from build123d import *

# Parameters (mm, degrees)
F0_R      = 23.0505
F0_R_2    = 16.7005
F1_DEPTH  = 50.8
F2_R      = 23.0505
F3_DEPTH  = 25.4
F3_FACE_R = 23.0505
F4_DEPTH  = 7.62
F5_R      = 16.7005
F6_DEPTH  = 7.62


with BuildPart() as f1:
    # F0 (on Top) → F1 (new body)
    with BuildSketch(Plane.XY):
        Circle(F0_R)
        Circle(F0_R_2, mode=Mode.SUBTRACT)
    extrude(amount=F1_DEPTH)

    # F2 (on face) → F3 (join)
    with BuildSketch(Plane.XY.offset(50.8)):
        Circle(F2_R)
    extrude(amount=F3_DEPTH)

    # F3_face (on face) → F4 (join)
    with BuildSketch(Plane.XY.offset(76.2)):
        Circle(F3_FACE_R)
    extrude(amount=F4_DEPTH)

    # F5 (on face) → F6 (cut)
    with BuildSketch(Plane.XY.offset(83.82)):
        Circle(F5_R)
    extrude(amount=-F6_DEPTH, mode=Mode.SUBTRACT)


solid = f1.part
The listing builds one solid part. Answer for the finished solid, in the listing's coordinates (mm). A direction names the side the tool comes from. Give positions to 0.01 mm unless a question says otherwise; leave off trailing zeros. Write each loop counter-clockwise with the first axis right and the second up, starting at its lowest first coordinate (ties: lowest second). Pieces come first, ordered by that corner, then holes.
Item 1: Which of the six approach directions +Z, -Z, +X, -X, +Y, -Y give full straight-line access (tool end or side, diameter ignored) to faces 4 (the cylindrical face through (-3.62, -16.303, 25.044)), 5 (the cylindrical face through (-3.62, -16.303, 80.063)), 6 (the flat face through (12, 12, 0))?
Item 2: Section C-C, the plane z = 14.5 is taken. Write down the section's boundary in (x, y).
Item 3: Find the intervals of material crossed by line 1 along Y through (x, z) = (0, 79); line 2 along Z through (x, y) = (-0.5, -1); line 3 along Y through (x, z) = (-7, 38), in increasing order.
Item 4: Determine the mould class of faces 1 (the cylindrical face through (-5, -22.5, 41.3)), 2 (the flat face through (12, 12, 83.82)), 3 (the flat face through (0, 0, 50.8)) for opening direction Y: released by +Y, released by -Y, zero draft, split by the parting line, or undercut.
Item 5: Flat-ended cylindrical pins translate along their axes: P1, Ø10, axis at x = 1.5, y = -7.5, coming from the -Z side; P2, Ø2, axis at x = -7.5, z = 10, coming from the -Y side; P3, Ø4, axis at y = -12.5, z = 39.5, coming from the -X side. Find the tip coordinate at first contact, or state that the pin passes through.
Item 6: Section D-D, the plane z = 70.5 is taken. Write down the section's boundary in (x, y), plus the area to 3 significant figures.
Item 7: Section A-A, the plane x = 0 is taken. Write down the section's boundary in (y, z).
Completed:
1. face 4: -Z
1. face 5: +Z
1. face 6: -Z, +X, -X, +Y, -Y
2. outline: circle Ø46.1 at (0, 0); hole circle Ø33.4 at (0, 0)
3. line 1: y = -23.05 to -16.7, 16.7 to 23.05
3. line 2: z = 50.8 to 76.2
3. line 3: y = -21.96 to -15.16, 15.16 to 21.96
4. face 1: split by the parting line
4. face 2: zero draft
4. face 3: undercut
5. P1: stops at z = 50.8
5. P2: stops at y = -22.12
5. P3: stops at x = -20.52
6. outline: circle Ø46.1 at (0, 0)
6. area: 1,670 mm2
7. outline: (-23.05, 0) - (-16.7, 0) - (-16.7, 50.8) - (16.7, 50.8) - (16.7, 0) - (23.05, 0) - (23.05, 83.82) - (16.7, 83.82) - (16.7, 76.2) - (-16.7, 76.2) - (-16.7, 83.82) - (-23.05, 83.82) - close
